Geometry check sheet. Reference: the model listing, model coordinates, mm. A direction names the side the tool comes from. Give positions to 0.01 mm unless a question says otherwise; leave off trailing zeros. Order: outer loops, then holes, each group sorted by start corner. A loop starts at its lowest first (then second) coordinate and runs counter-clockwise, first axis right, second up. Notation, with made-up numbers: M 26.5,58 L 83.5,58 A21 cw 83.5,86 Z; hole C -15,56.25 d1. An arc over 180 degrees is marked long. Put each result on its own line as item: value. Start each with the question number.
Q1. Access from +Z, -Z, +X, -X, +Y, -Y to the whole of each face (thin tool, end or side, straight path). Record for faces 1 (the cylindrical face through (-4.906, 2.114, -1.089)), 2 (the cylindrical face through (26.145, 1.014, 4.123)), 3 (the flat face through (-1.1, 3, 1.1)).
Q2. Material ranges on L1, parallel to X at y = 3.25, z = 0 (3 decimals); L2, parallel to Y at x = 8.5, z = 2.25; L3, parallel to X at y = 2.3, z = -1, recorded low to high.
Q3. Mould release check, pull along X, two halves, no side actions. Record for faces 4 (the flat face through (12, 1, 5.025)), 5 (the conical face through (-0.34, 1.85, -2.58)), 6 (the cylindrical face through (23.02, 1.01, -1.56)): +X half, -X half, draft (parallel to the pull), parting line (faces both ways), or undercut.
Q4. Section check D-D on x = 21.5. Record the cut outline in (y, z) (3 decimals), then the cut area to 3 significant figures.
Q5. Section check C-C on x = 9.5. Record the cut outline in (y, z) (3 decimals), then the cut area to 3 significant figures.
Q6. Section check B-B on z = 0. Record the cut outline in (x, y) (3 decimals), then the cut area to 3 significant figures.
Q7. Go/stop test with a flat-tipped pin: pin 1 (3 mm diameter, centred on x = 15, z = -3, fed in from -Y). Record where the tip stops, or that it passes through.
Q8. Section check A-A on y = 0.65. Record the cut outline in (x, z) (3 decimals), then the cut area to 3 significant figures.
```python
from build123d import *

# Parameters (mm, degrees)
SKETCH1_R           = 5.025
SKETCH1_R_2         = 2.025
BOSS_EXTRUDE1_DEPTH = 3
SKETCH2_W           = 27
SKETCH2_H           = 10.05
BOSS_EXTRUDE2_DEPTH = 2
SKETCH3_R           = 15
CUT_EXTRUDE1_DEPTH  = 2
FILLET1_R           = 3
SKETCH4_R           = 2.5
CUT_EXTRUDE2_DEPTH  = 10
CUT_EXTRUDE2_DRAFT  = 5
SKETCH5_R           = 5.025
BOSS_EXTRUDE3_DEPTH = 0.5
SKETCH6_R           = 1.4
CUT_EXTRUDE3_DEPTH  = 0.5


with BuildPart() as part:
    # Sketch1 → Boss-Extrude1 (new body)
    with BuildSketch(Plane(origin=(0, 0, 0), x_dir=(1, 0, 0), z_dir=(0, 1, 0))):
        with Locations(Location((0, 0, 0), (0, 0, 270))):
            Circle(SKETCH1_R)
        with Locations(Location((0, 0, 0), (0, 0, 270))):
            Circle(SKETCH1_R_2, mode=Mode.SUBTRACT)
    extrude(amount=BOSS_EXTRUDE1_DEPTH)

    # Sketch2 → Boss-Extrude2 (add)
    with BuildSketch(Plane.XZ):
        with Locations((13.5, 0)):
            Rectangle(SKETCH2_W, SKETCH2_H)
    extrude(amount=-BOSS_EXTRUDE2_DEPTH)

    # Sketch3 → Cut-Extrude1 (cut)
    with BuildSketch(Plane(origin=(0, 2, 0), x_dir=(1, 0, 0), z_dir=(0, 1, 0))):
        with Locations((32.816228029, 12.917418084)):
            Circle(SKETCH3_R)
    extrude(amount=-CUT_EXTRUDE1_DEPTH, mode=Mode.SUBTRACT)

    # Fillet1
    fillet1_edges = [part.edges().sort_by_distance(p)[0] for p in [
        (27, 1, 5.025),
    ]]
    fillet(fillet1_edges, radius=FILLET1_R)


with BuildPart() as cut_extrude2_tool:
    # Sketch4 → Cut-Extrude2 (with draft: the straight prism first)
    with BuildSketch(Plane(origin=(0, 3, 0), x_dir=(1, 0, 0), z_dir=(0, 1, 0))):
        Circle(SKETCH4_R)
    extrude(amount=-CUT_EXTRUDE2_DEPTH)
    # Cut-Extrude2: the draft: its side faces are tilted about the plane it starts from
    cut_extrude2_sides = [cut_extrude2_tool.faces().sort_by_distance(p)[0] for p in [
        (-2.5, -2, 0),
    ]]
    draft(cut_extrude2_sides, Plane(origin=(0, 3, 0), x_dir=(1, 0, 0), z_dir=(0, 1, 0)), CUT_EXTRUDE2_DRAFT)


with BuildPart() as part_1:
    add(part.part)

    # Cut-Extrude2: cut by cut_extrude2_tool
    add(cut_extrude2_tool.part, mode=Mode.SUBTRACT)

    # Sketch5 → Boss-Extrude3 (add)
    with BuildSketch(Plane(origin=(0, 3, 0), x_dir=(1, 0, 0), z_dir=(0, 1, 0))):
        with Locations(Location((0, 0, 0), (0, 0, 270))):
            Circle(SKETCH5_R)
    extrude(amount=BOSS_EXTRUDE3_DEPTH)

    # Sketch6 → Cut-Extrude3 (cut)
    with BuildSketch(Plane.XZ.offset(-3)):
        with Locations(Location((0, 0, 0), (0, 0, 270))):
            Circle(SKETCH6_R)
    extrude(amount=-CUT_EXTRUDE3_DEPTH, mode=Mode.SUBTRACT)


solid = part_1.part
```
Results found:
1. face 1: +Y
1. face 2: +Z, +X, +Y, -Y
1. face 3: -Y
2. L1: x = -5.025 to -1.4, 1.4 to 5.025
2. L2: y = 0 to 2
2. L3: x = -4.92 to -2.36, 2.36 to 4.92
3. face 4: draft
3. face 5: undercut
3. face 6: +X half
4. outline: M 0,-3.071 L 2,-3.071 L 2,5.025 L 0,5.025 Z
4. area: 16.2 mm^2
5. outline: M 0,-5.025 L 2,-5.025 L 2,5.025 L 0,5.025 Z
5. area: 20.1 mm^2
6. outline: M -5.025,0 L -2.762,0 L -2.5,3 L -1.4,3 L -1.4,3.5 L -5.025,3.5 Z; M 1.4,3 L 2.5,3 L 2.762,0 L 25.191,0 L 25.191,2 L 5.025,2 L 5.025,3.5 L 1.4,3.5 Z
6. area: 58.3 mm^2
7. pin 1: stops at y = 0
8. outline: M 0,-5.025 L 20.06,-5.025 A15 cw 27,0.909 L 27,2.025 A3 ccw 24,5.025 L 0,5.025 A5.025 ccw Z; hole C 0,0 d5.411
8. area: 261 mm^2
